Verification items for this drawing (mm, ordinates from the low corner). Give positions to 0.01 mm unless a question says otherwise; leave off trailing zeros. Write each loop counter-clockwise with the first axis right and the second up, starting at its lowest first coordinate (ties: lowest second). Pieces come first, ordered by that corner, then holes. Notation, with made-up numbers: (85, 27) -> (113, 27) arc R8 cw to (113, 39) -> close; hole circle Ø10 at (-2.5, 15.5). An arc over 180 degrees is marked (long way). Write item = value, one per line.
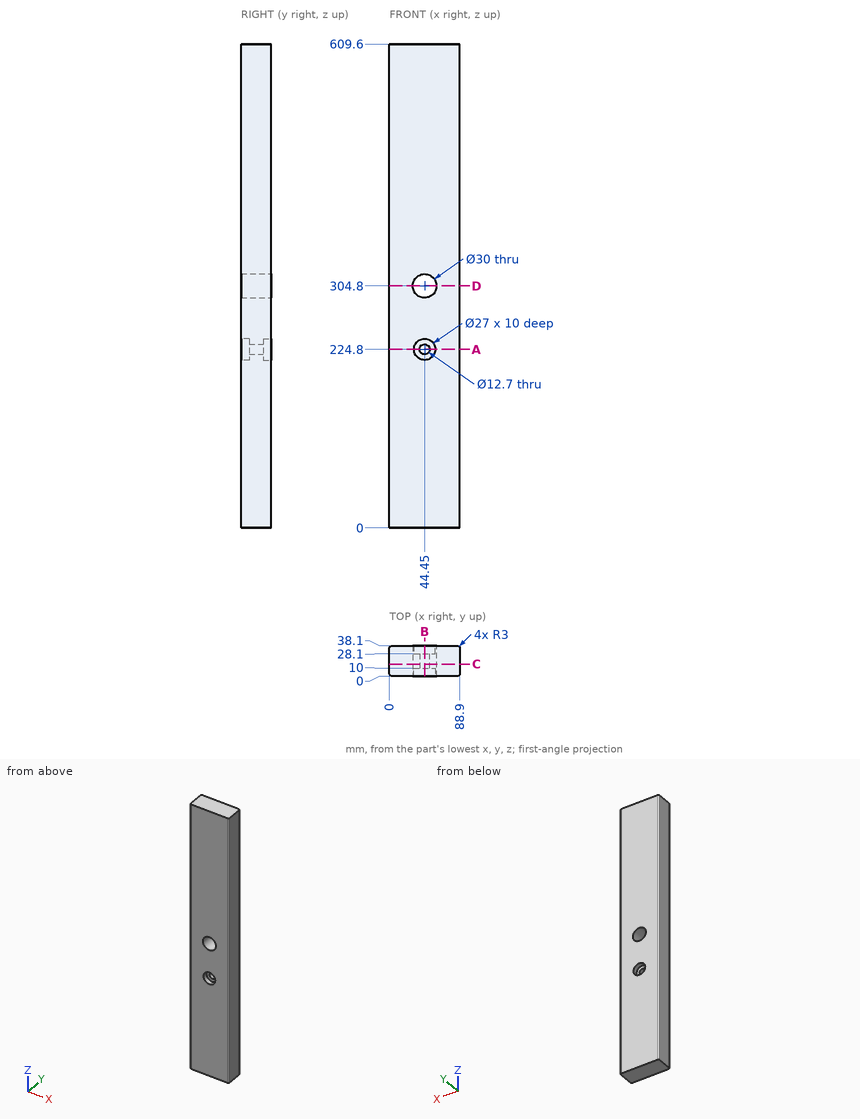
Item 1: Go/stop test with flat-tipped pins: P1, Ø24.5, axis at x = 44.45, z = 224.8, coming from the -Y side; P2, Ø11.5, axis at x = 44.45, z = 224.8, coming from the +Y side; P3, Ø8, axis at x = 41.5, z = 221, coming from the +Y side. Record where each tip stops, or that it passes through.
Response values:
P1 = 10
P2 = through
P3 = 28.1
Item 2: Sectioned sample at D-D on z = 304.8. Record the cut outline in (x, y).
Response values:
outline = (0, 3) arc R3 ccw to (3, 0) -> (29.45, 0) -> (29.45, 38.1) -> (3, 38.1) arc R3 ccw to (0, 35.1) -> close; (59.45, 0) -> (85.9, 0) arc R3 ccw to (88.9, 3) -> (88.9, 35.1) arc R3 ccw to (85.9, 38.1) -> (59.45, 38.1) -> close
Item 3: Sectioned sample at A-A on z = 224.8. Record the cut outline in (x, y).
Response values:
outline = (0, 3) arc R3 ccw to (3, 0) -> (30.95, 0) -> (30.95, 10) -> (38.1, 10) -> (38.1, 28.1) -> (30.95, 28.1) -> (30.95, 38.1) -> (3, 38.1) arc R3 ccw to (0, 35.1) -> close; (50.8, 10) -> (57.95, 10) -> (57.95, 0) -> (85.9, 0) arc R3 ccw to (88.9, 3) -> (88.9, 35.1) arc R3 ccw to (85.9, 38.1) -> (57.95, 38.1) -> (57.95, 28.1) -> (50.8, 28.1) -> close
Item 4: Sectioned sample at C-C on y = 15. Record the cut outline in (x, z).
Response values:
outline = (0, 0) -> (88.9, 0) -> (88.9, 609.6) -> (0, 609.6) -> close; hole circle Ø30 at (44.45, 304.8); hole circle Ø12.7 at (44.45, 224.8)
Item 5: Material ranges on line 1 (Z direction, x = 44.45, y = 5.75); line 2 (Z direction, x = 44.45, y = 22.25); line 3 (Z direction, x = 36, y = 24.5), recorded low to high.
Response values:
line_1 = 0 to 211.3, 238.3 to 289.8, 319.8 to 609.6
line_2 = 0 to 218.45, 231.15 to 289.8, 319.8 to 609.6
line_3 = 0 to 292.41, 317.19 to 609.6
Item 6: Sectioned sample at B-B on x = 44.45. Record the cut outline in (y, z), then the cut area to 3 significant figures.
Response values:
outline = (0, 0) -> (38.1, 0) -> (38.1, 211.3) -> (28.1, 211.3) -> (28.1, 218.45) -> (10, 218.45) -> (10, 211.3) -> (0, 211.3) -> close; (0, 238.3) -> (10, 238.3) -> (10, 231.15) -> (28.1, 231.15) -> (28.1, 238.3) -> (38.1, 238.3) -> (38.1, 289.8) -> (0, 289.8) -> close; (0, 319.8) -> (38.1, 319.8) -> (38.1, 609.6) -> (0, 609.6) -> close
area = 21,300 mm^2
